Drawing for the job (mm, zero at the part's lowest x, y, z). A direction names the side the tool comes from. Give positions to 0.01 mm unless a question says otherwise; leave off trailing zeros. Write each loop counter-clockwise with the first axis right and the second up, starting at its lowest first coordinate (ties: lowest second). Pieces come first, ordered by that corner, then holes. Notation, with made-up numbers: M 9,-30 L 61,-30 A18 cw 61,-19 Z; hole C 44,19.25 d11. An arc over 180 degrees is marked long. Use a Markdown table: item, result. Add a question column.
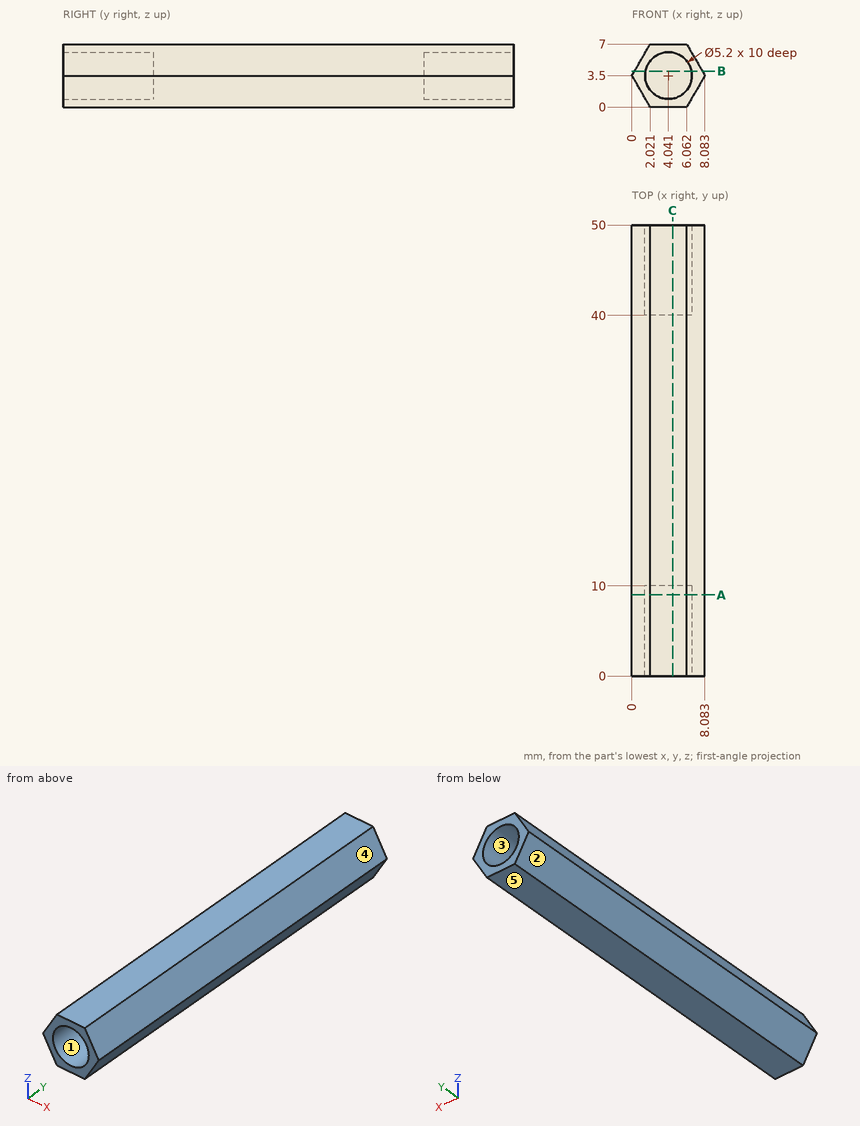
1. Cut at C-C (x = 4.5). Write the cut outline in (y, z).
2. Mould opens along X. For the marked faces 3, 4 and 5 say: released by +X, released by -X, zero draft, split by the parting line, or undercut.
3. Cut at B-B (z = 4). Write the cut outline in (x, y) (1 decimal), then the cut area to 3 significant figures.
4. Tool access for the marked faces 1 and 2: list every direction of +Z, -Z, +X, -X, +Y, -Y with a clear straight run to the whole face (end or side of a thin tool).
5. Cut at A-A (y = 9). Write the cut outline in (x, z), then the cut area to 3 significant figures.
6. Drill centre lines: probe 1 along X at (y, z) = (45.5, 3.5); probe 2 along Y at (x, z) = (3.25, 5.75); probe 3 along Z at (x, y) = (6.25, 41) (1 decimal). Where is each one in solid material? Low to high. Write a range as [from, to].
7. Flat gauge pins, fed straight in: pin 1 (3 mm diameter, centred on x = 4.04, z = 3.5, fed in from +Y); pin 2 (2.5 mm diameter, centred on x = 3, z = 4, fed in from -Y). Where does each tip first touch, or does it go through?
A:
| question | item | result |
|---|---|---|
| 1 | outline | M 0,0 L 50,0 L 50,0.94 L 40,0.94 L 40,6.06 L 50,6.06 L 50,7 L 0,7 L 0,6.06 L 10,6.06 L 10,0.94 L 0,0.94 Z |
| 2 | face 3 | undercut |
| 2 | face 4 | released by +X |
| 2 | face 5 | zero draft |
| 3 | outline | M 0.3,0 L 1.5,0 L 1.5,10 L 6.6,10 L 6.6,0 L 7.8,0 L 7.8,50 L 6.6,50 L 6.6,40 L 1.5,40 L 1.5,50 L 0.3,50 Z |
| 3 | area | 273 mm² |
| 4 | face 1 | -Y |
| 4 | face 2 | -Z, -X, +Y, -Y |
| 5 | outline | M 0,3.5 L 2.02,0 L 6.06,0 L 8.08,3.5 L 6.06,7 L 2.02,7 Z; hole C 4.04,3.5 d5.2 |
| 5 | area | 21.2 mm² |
| 6 | probe 1 | x = [0, 1.44], [6.64, 8.08] |
| 6 | probe 2 | y = [10, 40] |
| 6 | probe 3 | z = [0.3, 2.1], [4.9, 6.7] |
| 7 | pin 1 | stops at y = 40 |
| 7 | pin 2 | stops at y = 10 |
